CAD build for the part. Positions are in the model's coordinates, mm. A direction names the side the tool comes from. Give positions to 0.01 mm unless a question says otherwise; leave off trailing zeros. Order: outer loops, then holes, each group sorted by start corner. A loop starts at its lowest first (then second) coordinate and runs counter-clockwise, first axis right, second up.
Item 1: Band-saw the part on D-D on z = -9.5. Give the cut face in (x, y), plus the area to 3 significant figures.
Item 2: Flat gauge pins, fed straight in: P1, Ø2, axis at x = -1, y = -8, coming from the -Z side; P2, Ø1.5, axis at x = 5, y = -2, coming from the +Z side; P3, Ø2, axis at y = -3, z = -6.5, coming from the +X side (3 decimals); P4, Ø2.5, axis at x = 5.03, z = 0, coming from the +Y side. Where does each tip first touch, or does it go through?
Item 3: Band-saw the part on B-B on x = -4.25. Give the cut face in (y, z).
Item 4: Band-saw the part on C-C on z = -1. Give the cut face in (x, y), plus the area to 3 significant figures.
Item 5: Which spindle directions (+Z, -Z, +X, -X, +Y, -Y) get a long thin tool onto all of the face, cutting with end or side? Do faces 1 (the cylindrical face through (-1.5, -4.93, 0.07)), 2 (the flat face through (2.775, -1.479, 1.328)), 3 (the flat face through (-0.1, -5, 10.2)). Say none if no direction does.
Item 6: Two-plate mould, pull along Z, no slides. Class faces 4 (the flat face through (2.754, -1.479, -1.292)), 5 (the cylindrical face through (-2.17, -7.46, -9.76)), 6 (the cylindrical face through (-6.482, -6.451, 0.064)), 7 (the flat face through (0, 0, -3)): released by +Z, released by -Z, zero draft, split by the parting line, or undercut.
Item 7: Band-saw the part on A-A on y = -1. Give the cut face in (x, z).
Item 8: Wall check: L1, parallel to X at y = -4.75, z = 0.5; L2, parallel to X at y = -7, z = -0.5; L3, parallel to Y at x = 6, z = -2.5. Give the ranges that are in metal, low to high.
```python
from build123d import *

# Parameters (mm, degrees)
F0_R     = 12.5
F0_R_2   = 10
F1_DEPTH = 5
F0_R_3   = 1.5
F2_DEPTH = 10
F3_R     = 1.45
F4_DEPTH = 25
F5_DEPTH = 25
F6_DEPTH = 3


with BuildPart() as f1:
    # F0 (on Front) → F1 (new body)
    with BuildSketch(Plane.XZ):
        Circle(F0_R)
        Circle(F0_R_2, mode=Mode.SUBTRACT)
    extrude(amount=F1_DEPTH)

    # F0 (on Front) → F2 (join)
    with BuildSketch(Plane.XZ):
        Circle(F0_R_2)
        Circle(F0_R_3, mode=Mode.SUBTRACT)
    extrude(amount=F2_DEPTH)

    # F3 (on Front) → F4 (cut)
    with BuildSketch(Plane.XZ):
        with Locations((-5.033278, 0)):
            Circle(F3_R)
    extrude(amount=F4_DEPTH, mode=Mode.SUBTRACT)

    # F3 (on Front) → F5 (cut)
    with BuildSketch(Plane.XZ):
        with Locations((5.033278, 0)):
            Circle(F3_R)
    extrude(amount=F5_DEPTH, mode=Mode.SUBTRACT)

    # F3 (on Front) → F6 (cut)
    with BuildSketch(Plane.XZ):
        Polygon((-6.545778, -2.619727), (-3.520778, -2.619727), (-2.008278, 0), (-3.520778, 2.619727), (-6.545778, 2.619727), (-8.058278, 0), align=None)
        with Locations((-5.033278, 0)):
            Circle(F3_R, mode=Mode.SUBTRACT)
        Polygon((6.545778, -2.619727), (8.058278, 0), (6.545778, 2.619727), (3.520778, 2.619727), (2.008278, 0), (3.520778, -2.619727), align=None)
        with Locations((5.033278, 0)):
            Circle(F3_R, mode=Mode.SUBTRACT)
    extrude(amount=F6_DEPTH, mode=Mode.SUBTRACT)


solid = f1.part
```
The answers:
1. outline: (-8.12, -5) - (-3.12, -5) - (-3.12, -10) - (3.12, -10) - (3.12, -5) - (8.12, -5) - (8.12, 0) - (-8.12, 0) - close
1. area: 112 mm2
2. P1: stops at z = -10
2. P2: stops at z = 11.76
2. P3: stops at x = 11.225
2. P4: passes through
3. outline: (-10, -9.05) - (-5, -9.05) - (-5, -11.76) - (0, -11.76) - (0, -2.62) - (-3, -2.62) - (-3, -1.22) - (-10, -1.22) - close; (-10, 1.22) - (-3, 1.22) - (-3, 2.62) - (0, 2.62) - (0, 11.76) - (-5, 11.76) - (-5, 9.05) - (-10, 9.05) - close
4. outline: (-12.46, -5) - (-9.95, -5) - (-9.95, -10) - (-6.08, -10) - (-6.08, -3) - (-7.48, -3) - (-7.48, 0) - (-12.46, 0) - close; (-3.98, -10) - (-1.12, -10) - (-1.12, 0) - (-2.59, 0) - (-2.59, -3) - (-3.98, -3) - close; (1.12, -10) - (3.98, -10) - (3.98, -3) - (2.59, -3) - (2.59, 0) - (1.12, 0) - close; (6.08, -10) - (9.95, -10) - (9.95, -5) - (12.46, -5) - (12.46, 0) - (7.48, 0) - (7.48, -3) - (6.08, -3) - close
4. area: 143 mm2
5. face 1: +Y, -Y
5. face 2: +Y
5. face 3: -Y
6. face 4: undercut
6. face 5: split by the parting line
6. face 6: undercut
6. face 7: zero draft
7. outline: circle Ø25 at (0, 0); hole (-8.06, 0) - (-6.55, -2.62) - (-3.52, -2.62) - (-2.01, 0) - (-3.52, 2.62) - (-6.55, 2.62) - close; hole circle Ø3 at (0, 0); hole (2.01, 0) - (3.52, -2.62) - (6.55, -2.62) - (8.06, 0) - (6.55, 2.62) - (3.52, 2.62) - close
8. L1: x = -12.49 to -6.39, -3.67 to -1.41, 1.41 to 3.67, 6.39 to 12.49
8. L2: x = -9.99 to -6.39, -3.67 to -1.41, 1.41 to 3.67, 6.39 to 9.99
8. L3: y = -10 to -3
